from build123d import *

# Parameters (mm, degrees)
F0_W     = 60
F0_H     = 60
F1_DEPTH = 70
F3_DEPTH = 70.001
F5_DEPTH = 30.001


with BuildPart() as f1:
    # F0 (on Top) → F1 (new body)
    with BuildSketch(Plane.XY):
        Rectangle(F0_W, F0_H)
    extrude(amount=F1_DEPTH)

    # F2 (on face) → F3 (cut, through all)
    with BuildSketch(Plane.XY.offset(70)):
        with BuildLine():
            ThreePointArc((0, 30), (21.213203, 21.213203), (30, 0))
            Line((30, 0), (30, 30))
            Line((30, 30), (0, 30))
        make_face()
        with BuildLine():
            ThreePointArc((-30, 0), (-21.213203, 21.213203), (0, 30))
            Line((0, 30), (-30, 30))
            Line((-30, 30), (-30, 0))
        make_face()
    extrude(amount=-F3_DEPTH, mode=Mode.SUBTRACT)

    # F4 (on Right) → F5 (cut, through all)
    with BuildSketch(Plane.YZ):
        Polygon((30, 0), (29.520035, 69.998355), (0, 0), align=None)
    extrude(amount=-F5_DEPTH, mode=Mode.SUBTRACT)


solid = f1.part
Part model, mm, in its own coordinate system. A direction names the side the tool comes from. Coordinates: 2 decimals unless noted, no trailing zeros. Loops run counter-clockwise (first coordinate to the right, second up) from the corner with the lowest first, then second, coordinate; pieces in that order, holes last. Notation, with made-up numbers: (-22, 34.25) - (-10, 34.25) arc R20 ccw to (-10, 55.25) - close; hole circle Ø8 at (54, 41.25). An arc over 180 degrees is marked (long way). Write each question's results on one line, items separated by ' | '. Start each with the question number.
Q1. Which spindle directions (+Z, -Z, +X, -X, +Y, -Y) get a long thin tool onto all of the face, cutting with end or side? Do faces 1 (the flat face through (0, 21, 20)), 2 (the flat face through (0, -30, 35)). Say none if no direction does.
Q2. Slice it at D-D on z = 14. Give the cut face in (x, y).
Q3. Slice it at C-C on x = -9.5. Give the cut face in (y, z), and give its area (3 significant figures).
Q4. Probe line 1 along X through (y, z) = (0.5, 41.5); line 2 along Y through (x, z) = (-12.5, 10.5); line 3 along X through (y, z) = (24, 20). List the from-to ranges inside material, lowest first.
Q5. Drop flat-ended pins along their axis: pin 1 Ø5 at (y, z) = (9, 17) entering from +X; pin 2 Ø8 at (y, z) = (15.5, 9) entering from -X; pin 3 Ø12 at (x, z) = (0.5, 15) entering from +Y; pin 4 Ø10 at (x, z) = (-23, 17) entering from +Y. Give the stop position or say it passes through.
Q6. Slice it at B-B on y = 11.5. Give the cut face in (x, z), and give its area (3 significant figures).
Q7. Slice it at A-A on z = 33. Give the cut face in (x, y).
Answer:
1) face 1: -Z, -X | face 2: +Z, -Z, +X, -X, -Y
2) outline: (-30, -30) - (30, -30) - (30, 0) arc R30 ccw to (0, 30) arc R30 ccw to (-2.4, 29.9) - (0, 29.9) - (0, 5.9) - (-29.41, 5.9) arc R30 ccw to (-30, 0) - close
3) outline: (-30, 0) - (0, 0) - (28.46, 67.48) - (28.46, 70) - (-30, 70) - close | area: 3,130 mm2
4) line 1: x = -30 to 30 | line 2: y = -30 to 4.43 | line 3: x = 0 to 18
5) pin 1: stops at x = 29.29 | pin 2: stops at x = 0 | pin 3: stops at y = 30 | pin 4: stops at y = 9.28
6) outline: (-27.71, 27.27) - (0, 27.27) - (0, 0) - (27.71, 0) - (27.71, 70) - (-27.71, 70) - close | area: 3,120 mm2
7) outline: (-30, -30) - (30, -30) - (30, 0) arc R30 ccw to (0, 30) arc R30 ccw to (-3.68, 29.77) - (0, 29.77) - (0, 13.92) - (-26.58, 13.92) arc R30 ccw to (-30, 0) - close
